Job drawing, mm, ordinate dimensions from the low corner. One solid piece. Round coordinates to 2 decimals unless told otherwise and drop trailing zeros. Loops run counter-clockwise (first coordinate to the right, second up) from the corner with the lowest first, then second, coordinate; pieces in that order, holes last.
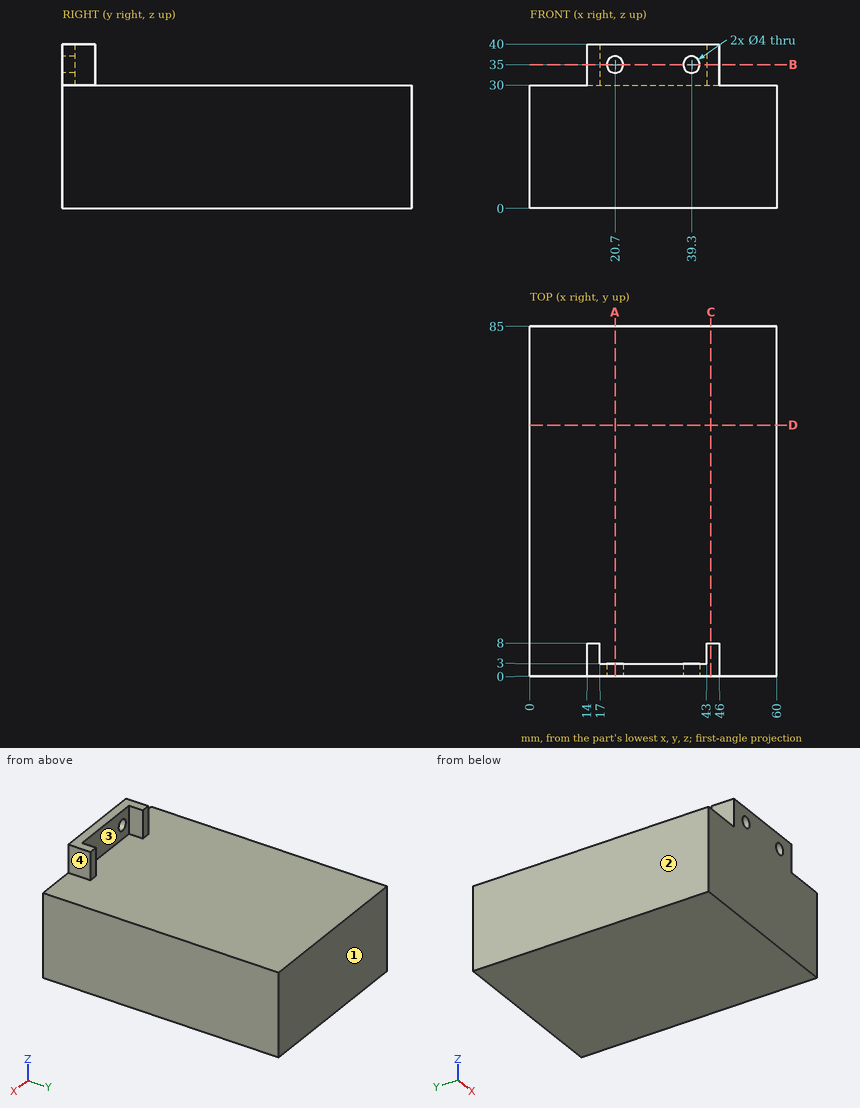
(1) Slice it at A-A on x = 20.7. List the corners of the cut face in (y, z), plus the area to 3 significant figures.
Responses:
outline: (0, 0) - (85, 0) - (85, 30) - (3, 30) - (3, 33) - (0, 33) - close; (0, 37) - (3, 37) - (3, 40) - (0, 40) - close
area: 2,570 mm2
(2) Pin check, flat tips, straight feed: P1, Ø1.5, axis at x = 47.5, y = 43, coming from the +Z side; P2, Ø2, axis at x = 16.5, z = 33, coming from the +Y side; P3, Ø4, axis at y = 5.5, z = 36, coming from the -X side. Stop position of each tip, or through.
Responses:
P1: stops at z = 30
P2: stops at y = 8
P3: stops at x = 14
(3) Pull direction X, two halves, no side cores. Call the marked faces 1, 2, 3 and 4: +X half, -X half, draft (parallel to the pull), parting line (faces both ways), or undercut.
Responses:
face 1: draft
face 2: -X half
face 3: undercut
face 4: +X half
(4) Slice it at B-B on z = 35. List the corners of the cut face in (x, y).
Responses:
outline: (14, 0) - (18.7, 0) - (18.7, 3) - (17, 3) - (17, 8) - (14, 8) - close; (22.7, 0) - (37.3, 0) - (37.3, 3) - (22.7, 3) - close; (41.3, 0) - (46, 0) - (46, 8) - (43, 8) - (43, 3) - (41.3, 3) - close
(5) Slice it at C-C on x = 44. List the corners of the cut face in (y, z).
Responses:
outline: (0, 0) - (85, 0) - (85, 30) - (8, 30) - (8, 40) - (0, 40) - close
(6) Probe line 1 (X direction, y = 2, z = 35); line 2 (Z direction, x = 39, y = 2); line 3 (X direction, y = 5.5, z = 34). List the from-to ranges inside material, lowest first.
Responses:
line 1: x = 14 to 18.7, 22.7 to 37.3, 41.3 to 46
line 2: z = 0 to 33.02, 36.98 to 40
line 3: x = 14 to 17, 43 to 46
(7) Slice it at D-D on y = 61. List the corners of the cut face in (x, z), plus the area to 3 significant figures.
Responses:
outline: (0, 0) - (60, 0) - (60, 30) - (0, 30) - close
area: 1,800 mm2
